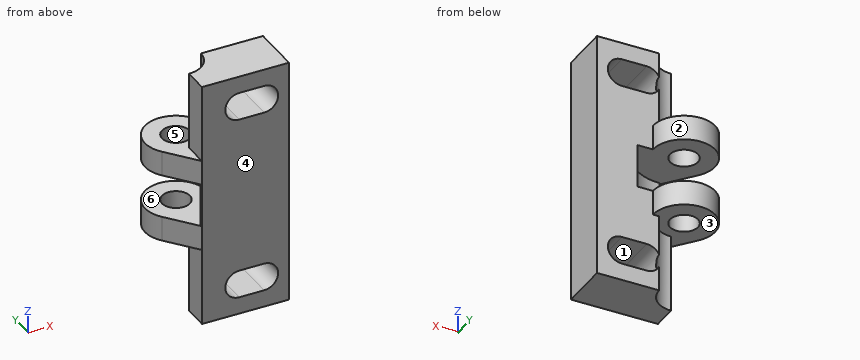
from build123d import *

# Parameters (mm, degrees)
SKETCH1_W               = 13
SKETCH1_H               = 15
BOSS_EXTRUDE1_DEPTH     = 8
BOSS_EXTRUDE2_DEPTH     = 4
SKETCH6_W               = 14
SKETCH6_H               = 40
BOSS_EXTRUDE3_DEPTH     = 8
SKETCH3_R               = 7.5
CUT_EXTRUDE1_DEPTH      = 7
CUT_EXTRUDE2_DEPTH      = 36.344730866
CUT_EXTRUDE2_DEPTH_BACK = 36.344730866
SKETCH4_R               = 2.25
SKETCH7_R               = 4
CUT_EXTRUDE3_DEPTH      = 36.344730866


with BuildPart() as part:
    # Sketch1 → Boss-Extrude1 (new body)
    with BuildSketch(Plane(origin=(0, 0, 0), x_dir=(1, 0, 0), z_dir=(0, 1, 0))):
        with Locations((-6.5, 0)):
            Rectangle(SKETCH1_W, SKETCH1_H)
    extrude(amount=BOSS_EXTRUDE1_DEPTH)

    # Sketch2 → Boss-Extrude2 (add)
    with BuildSketch(Plane.XY.offset(7.5)):
        with BuildLine():
            Line((-16.903123749, 4.875), (-13, 0))
            Line((-13, 0), (-13, 3))
            ThreePointArc((-13, 3), (-10.834936491, 12.506939094), (-16.903123749, 4.875))
        make_face()
    boss_extrude2 = extrude(amount=-BOSS_EXTRUDE2_DEPTH)

    # Mirror1: Boss-Extrude2 across plane
    add(boss_extrude2.mirror(Plane.XY))

    # Sketch6 → Boss-Extrude3 (add)
    with BuildSketch(Plane.XZ):
        with Locations((-6, 0)):
            Rectangle(SKETCH6_W, SKETCH6_H)
        with BuildLine():
            Line((-7, 17.25), (-3, 17.25))
            ThreePointArc((-3, 17.25), (-0.75, 15), (-3, 12.75))
            Line((-3, 12.75), (-7, 12.75))
            ThreePointArc((-7, 12.75), (-9.25, 15), (-7, 17.25))
        make_face(mode=Mode.SUBTRACT)
        with BuildLine():
            Line((-7, -12.75), (-3, -12.75))
            ThreePointArc((-3, -12.75), (-0.75, -15), (-3, -17.25))
            Line((-3, -17.25), (-7, -17.25))
            ThreePointArc((-7, -17.25), (-9.25, -15), (-7, -12.75))
        make_face(mode=Mode.SUBTRACT)
    extrude(amount=-BOSS_EXTRUDE3_DEPTH)

    # Sketch3 → Cut-Extrude1 (cut)
    with BuildSketch(Plane.XY.offset(-3.5)):
        with Locations((-13, 8)):
            Circle(SKETCH3_R)
    extrude(amount=CUT_EXTRUDE1_DEPTH, mode=Mode.SUBTRACT)

    # Sketch4 → Cut-Extrude2 (cut, two sides: drawn at the far end of the back side and taken through both)
    with BuildSketch(Plane.XY.offset(7.5).offset(-CUT_EXTRUDE2_DEPTH_BACK)):
        with Locations((-13, 8)):
            Circle(SKETCH4_R)
    extrude(amount=CUT_EXTRUDE2_DEPTH + CUT_EXTRUDE2_DEPTH_BACK, mode=Mode.SUBTRACT)

    # Sketch7 → Cut-Extrude3 (cut, through all)
    with BuildSketch(Plane.XY.offset(7.5)):
        with Locations((-13, 8)):
            Circle(SKETCH7_R)
    cut_extrude3 = extrude(amount=CUT_EXTRUDE3_DEPTH, mode=Mode.SUBTRACT)

    # Mirror2: Cut-Extrude3 across plane
    add(cut_extrude3.mirror(Plane.XY), mode=Mode.SUBTRACT)


solid = part.part
Geometry check sheet. Reference: the model listing, model coordinates, mm. Face numbers are marked on the shaded views. A direction names the side the tool comes from. Round coordinates to 2 decimals unless told otherwise and drop trailing zeros. Loops run counter-clockwise (first coordinate to the right, second up) from the corner with the lowest first, then second, coordinate; pieces in that order, holes last. Notation, with made-up numbers: (1.5, -17.75) -> (57.5, -17.75) arc R31 ccw to (57.5, 6.25) -> close; hole circle Ø4 at (32, 22). An arc over 180 degrees is marked (long way). Answer as a JSON object with one key per item and string values. Group by question number.
Item 1: Thickness scan on line 1 along Z through (x, y) = (-6.5, 7.75); line 2 along Z through (x, y) = (-6.5, 1.25); line 3 along Z through (x, y) = (-11.25, 9.5). Record the ranges inside material, lowest first.
Item 2: Cross-section at B-B, the plane y = 9.25. Record the cut outline in (x, z), plus the area to 3 significant figures.
Item 3: Set-up check for the marked faces 1, 2 and 3: record each of +Z, -Z, +X, -X, +Y, -Y from which the full face is reachable in a straight line by a thin tool's end or side.
Item 4: Cross-section at C-C, the plane x = -16.25. Record the cut outline in (y, z).
Item 5: Cross-section at A-A, the plane z = 15. Record the cut outline in (x, y), plus the area to 3 significant figures.
Item 6: Cross-section at D-D, the plane x = -6.5. Record the cut outline in (y, z), plus the area to 3 significant figures.
Item 7: Release check for a two-part mould opening along Y. For the marked faces 4, 5 and 6 record: pulls with the +Y half, pulls with the -Y half, needs draft (parallel to the pull), parting line crosses it, or undercut.
Item 8: Depth check by flat-ended pin: pin 1 Ø5 at (x, z) = (-2.5, -3) entering from +Y; pin 2 Ø3 at (y, z) = (10.5, -12) entering from +X; pin 3 Ø4 at (y, z) = (9.5, -9) entering from +X; pin 4 Ø5 at (x, y) = (-13, 8) entering from -Z. Enter the tip coordinate at first touch or a pass-through.
Determined:
{
 "1": {"line 1": "z = -20 to -17.25, -12.75 to -3.5, 3.5 to 12.75, 17.25 to 20", "line 2": "z = -20 to -17.25, -12.75 to 12.75, 17.25 to 20", "line 3": "z = -7.5 to -3.5, 3.5 to 7.5"},
 "2": {"outline": "(-17.84, -7.5) -> (-14.87, -7.5) -> (-14.87, -3.5) -> (-17.84, -3.5) -> close; (-17.84, 3.5) -> (-14.87, 3.5) -> (-14.87, 7.5) -> (-17.84, 7.5) -> close; (-11.13, -7.5) -> (-8.16, -7.5) -> (-8.16, -3.5) -> (-11.13, -3.5) -> close; (-11.13, 3.5) -> (-8.16, 3.5) -> (-8.16, 7.5) -> (-11.13, 7.5) -> close", "area": "47.5 mm²"},
 "3": {"face 1": "+Y, -Y", "face 2": "+Z, -Z", "face 3": "-Z, -X, +Y"},
 "4": {"outline": "(4.06, -7.5) -> (11.8, -7.5) -> (11.8, -3.5) -> (4.06, -3.5) -> close; (4.06, 3.5) -> (11.8, 3.5) -> (11.8, 7.5) -> (4.06, 7.5) -> close"},
 "5": {"outline": "(-13, 0) -> (-9.25, 0) -> (-9.25, 6.61) arc R4 cw to (-13, 4) -> close; (-0.75, 0) -> (1, 0) -> (1, 8) -> (-0.75, 8) -> close", "area": "31.7 mm²"},
 "6": {"outline": "(0, -20) -> (8, -20) -> (8, -17.25) -> (0, -17.25) -> close; (0, -12.75) -> (8, -12.75) -> (8, -3.5) -> (4.26, -3.5) -> (4.26, 3.5) -> (8, 3.5) -> (8, 12.75) -> (0, 12.75) -> close; (0, 17.25) -> (8, 17.25) -> (8, 20) -> (0, 20) -> close", "area": "222 mm²"},
 "7": {"face 4": "pulls with the -Y half", "face 5": "undercut", "face 6": "needs draft"},
 "8": {"pin 1": "stops at y = 8", "pin 2": "passes through", "pin 3": "stops at x = 1", "pin 4": "stops at z = -7.5"}
}
